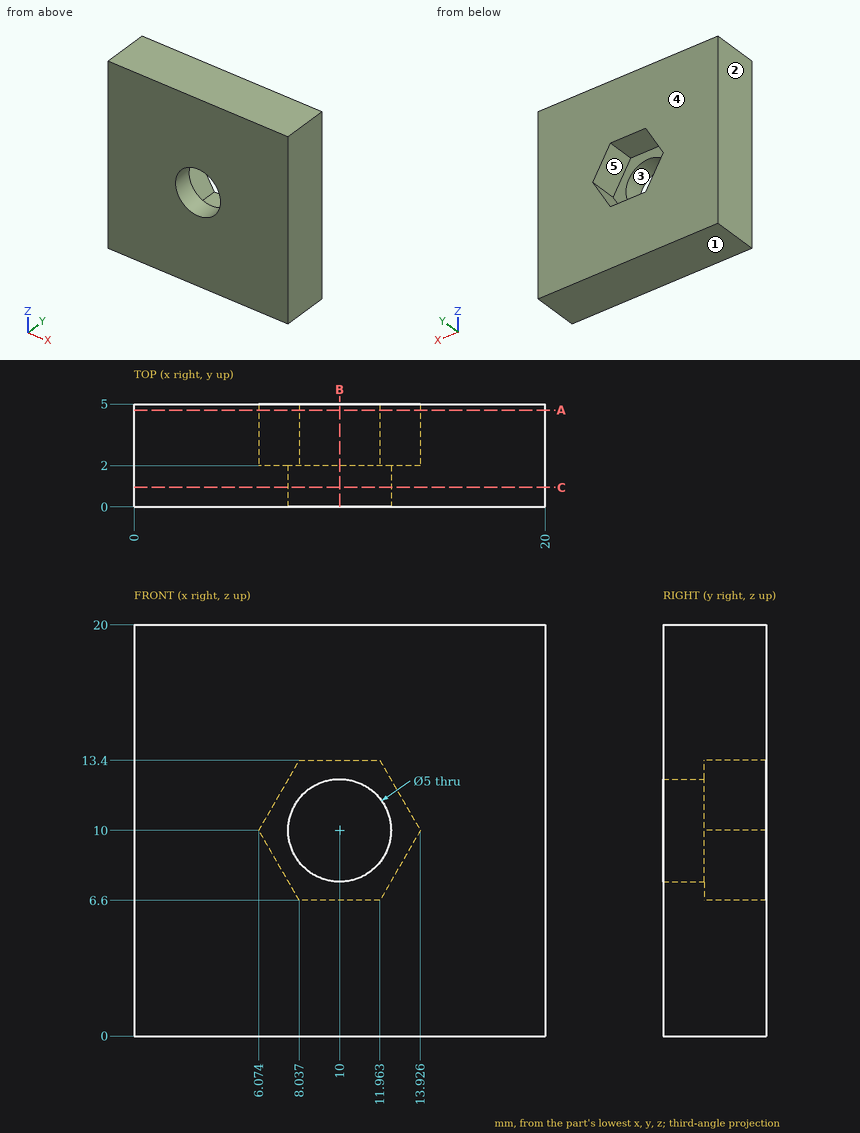
Drawing for the job (mm, zero at the part's lowest x, y, z). A direction names the side the tool comes from. Give positions to 0.01 mm unless a question says otherwise; leave off trailing zeros. Loops run counter-clockwise (first coordinate to the right, second up) from the corner with the lowest first, then second, coordinate; pieces in that order, holes last.
1) Band-saw the part on A-A on y = 4.7. List the corners of the cut face in (x, z).
Values follow:
outline: (0, 0) - (20, 0) - (20, 20) - (0, 20) - close; hole (6.07, 10) - (8.04, 6.6) - (11.96, 6.6) - (13.93, 10) - (11.96, 13.4) - (8.04, 13.4) - close
2) Band-saw the part on B-B on x = 10. List the corners of the cut face in (y, z), then the cut area to 3 significant figures.
Values follow:
outline: (0, 0) - (5, 0) - (5, 6.6) - (2, 6.6) - (2, 7.5) - (0, 7.5) - close; (0, 12.5) - (2, 12.5) - (2, 13.4) - (5, 13.4) - (5, 20) - (0, 20) - close
area: 69.6 mm2
3) Band-saw the part on C-C on y = 0.95. List the corners of the cut face in (x, z), then the cut area to 3 significant figures.
Values follow:
outline: (0, 0) - (20, 0) - (20, 20) - (0, 20) - close; hole circle Ø5 at (10, 10)
area: 380 mm2
4) Probe line 1 along Z through (x, y) = (10, 1.2); line 2 along Z through (x, y) = (11.5, 2.2). List the from-to ranges inside material, lowest first.
Values follow:
line 1: z = 0 to 7.5, 12.5 to 20
line 2: z = 0 to 6.6, 13.4 to 20
5) Drop a flat-ended pin along its axis: P1, Ø5.5, axis at x = 10, z = 9.5, coming from the +Y side. Give the stop position or say it passes through.
Values follow:
P1: stops at y = 2
6) Two-plate mould, pull along Z, no slides. Class the marked faces 1, 2 and 3: released by +Z, released by -Z, zero draft, split by the parting line, or undercut.
Values follow:
face 1: released by -Z
face 2: zero draft
face 3: undercut
7) 3-axis set-ups, long thin cutter, end or side, ignore diameter. For the marked faces 4 and 5: which of +Z, -Z, +X, -X, +Y, -Y reach the whole face in a straight line?
Values follow:
face 4: +Z, -Z, +X, -X, +Y
face 5: +Y
